```python
from build123d import *

# Parameters (mm, degrees)
SKETCH1_R               = 45
SKETCH1_R_2             = 6.2
BOSS_EXTRUDE1_DEPTH     = 7.5
SKETCH2_W               = 5.3
SKETCH2_H               = 10.6
CUT_EXTRUDE1_DEPTH      = 13
SKETCH3_R               = 3.25
CUT_EXTRUDE2_DEPTH      = 37.4
CUT_EXTRUDE2_DEPTH_BACK = 13
FILLET1_R               = 4


with BuildPart() as part:
    # Sketch1 → Boss-Extrude1 (new body, symmetric)
    with BuildSketch(Plane.XY):
        Circle(SKETCH1_R)
        Circle(SKETCH1_R_2, mode=Mode.SUBTRACT)
    extrude(amount=BOSS_EXTRUDE1_DEPTH, both=True)

    # Sketch2 → Cut-Extrude1 (cut)
    with BuildSketch(Plane.XY.offset(7.5)):
        with Locations((11.25, 0)):
            Rectangle(SKETCH2_W, SKETCH2_H)
    extrude(amount=-CUT_EXTRUDE1_DEPTH, mode=Mode.SUBTRACT)

    # Sketch3 → Cut-Extrude2 (cut, two sides)
    with BuildSketch(Plane(origin=(8.6, 0, 0), x_dir=(0, 0, -1), z_dir=(1, 0, 0))) as cut_extrude2_sk:
        Circle(SKETCH3_R)
    extrude(amount=CUT_EXTRUDE2_DEPTH, mode=Mode.SUBTRACT)
    extrude(cut_extrude2_sk.sketch, amount=-CUT_EXTRUDE2_DEPTH_BACK, mode=Mode.SUBTRACT)

    # Fillet1
    fillet1_edges = [part.edges().sort_by_distance(p)[0] for p in [
        (-45, 0, -7.5),
        (-45, 0, 7.5),
    ]]
    fillet(fillet1_edges, radius=FILLET1_R)


solid = part.part
```
Input: part model. Units: mm. Frame: model coordinates. A direction names the side the tool comes from. Round coordinates to 2 decimals unless told otherwise and drop trailing zeros. Loops run counter-clockwise (first coordinate to the right, second up) from the corner with the lowest first, then second, coordinate; pieces in that order, holes last. Notation, with made-up numbers: (-22, -37) -> (35, -37) arc R33 cw to (35, -8) -> close; hole circle Ø4 at (80, 87.25). An arc over 180 degrees is marked (long way). Use one line per item in the form item = value. Start each with the question number.
Item 1: Section query A-A on x = 0. Return the cut outline in (y, z), then the cut area to 3 significant figures.
Item 2: Section query C-C on z = 0.75. Return the cut outline in (x, y).
Item 3: Contact query for flat-ended pins moving along their axis: pin 1 Ø7.5 at (x, y) = (0, 0) entering from +Z; pin 2 Ø1.5 at (x, z) = (10, -1) entering from -Y; pin 3 Ø2 at (y, z) = (17.5, -3) entering from +X; pin 4 Ø6 at (x, z) = (12.5, -2) entering from +Y. Output: stop coordinate, or through.
Item 4: Mould query, pull axis Z, two halves, no side actions, for faces 1 (the face through (-1, -9, 7.5)), 2 (the face through (7.332, 2.197, 2.395)), 3 (the face through (9, 1, -7.5)). Classes: pulls with the +Z half, pulls with the -Z half, needs draft (parallel to the pull), parting line crosses it, or undercut.
Item 5: Set-up query: faces 4 (the face through (-6.194, 0.273, -0.105)), 5 (the face through (11, -5.3, 1)), 6 (the face through (29.232, -1.978, 2.579)). Return all of +Z, -Z, +X, -X, +Y, -Y with unobstructed straight access to the full face (end or side cutting, diameter ignored); none if empty.
Item 6: Material intervals for L1, parallel to Y at x = 0, z = -1; L2, parallel to Y at x = 36, z = 0; L3, parallel to Z at x = 7.25, y = 0, sorted ascending. Write a range as from..to.
Item 7: Section query B-B on y = 0. Return the cut outline in (x, z).
Ans:
q1.outline = (-45, -3.5) arc R4 ccw to (-41, -7.5) -> (-6.2, -7.5) -> (-6.2, 7.5) -> (-41, 7.5) arc R4 ccw to (-45, 3.5) -> close; (6.2, -7.5) -> (41, -7.5) arc R4 ccw to (45, -3.5) -> (45, 3.5) arc R4 ccw to (41, 7.5) -> (6.2, 7.5) -> close
q1.area = 1,150 mm^2
q2.outline = (5.33, -3.16) arc R6.2 cw (long way) to (5.33, 3.16) -> (8.6, 3.16) -> (8.6, 5.3) -> (13.9, 5.3) -> (13.9, 3.16) -> (44.89, 3.16) arc R45 ccw (long way) to (44.89, -3.16) -> (13.9, -3.16) -> (13.9, -5.3) -> (8.6, -5.3) -> (8.6, -3.16) -> close
q3.pin_1 = through
q3.pin_2 = -44.04
q3.pin_3 = 41.87
q3.pin_4 = 43.99
q4.face_1 = pulls with the +Z half
q4.face_2 = undercut
q4.face_3 = pulls with the -Z half
q5.face_4 = +Z, -Z
q5.face_5 = +Z
q5.face_6 = +X
q6.L1 = -45..-6.2, 6.2..45
q6.L2 = -27..-3.25, 3.25..27
q6.L3 = -7.5..-3.25, 3.25..7.5
q7.outline = (-45, -3.5) arc R4 ccw to (-41, -7.5) -> (-6.2, -7.5) -> (-6.2, 7.5) -> (-41, 7.5) arc R4 ccw to (-45, 3.5) -> close; (6.2, -7.5) -> (41, -7.5) arc R4 ccw to (45, -3.5) -> (45, -3.25) -> (13.9, -3.25) -> (13.9, -5.5) -> (8.6, -5.5) -> (8.6, -3.25) -> (6.2, -3.25) -> close; (6.2, 3.25) -> (8.6, 3.25) -> (8.6, 7.5) -> (6.2, 7.5) -> close; (13.9, 3.25) -> (45, 3.25) -> (45, 3.5) arc R4 ccw to (41, 7.5) -> (13.9, 7.5) -> close
